Source: CAD feature listing. Evaluate the final solid. Frame: model axes, mm. Round coordinates to 2 decimals unless told otherwise and drop trailing zeros. Loops run counter-clockwise (first coordinate to the right, second up) from the corner with the lowest first, then second, coordinate; pieces in that order, holes last. Notation, with made-up numbers: M 57.25,-3 L 67.25,-3 A30 cw 67.25,36 Z; hole C 44.5,-4.75 d2. An arc over 180 degrees is marked long. Answer as a JSON object with one key per item and string values.
from build123d import *

# Parameters (mm, degrees)
KEYED_BACK_DEPTH   = 0.7
CUP_BLANK_SKETCH_R = 3.8
CUP_BLANK_DEPTH    = 3.3


with BuildPart() as part:
    # Keyed Back Sketch → Keyed Back (new body)
    with BuildSketch(Plane(origin=(0, -97, 0), x_dir=(-1, 0, 0), z_dir=(0, -1, 0))):
        with BuildLine():
            Line((29.790988145, 11.23573341), (33.83079012, 13.568114168))
            ThreePointArc((33.83079012, 13.568114168), (28.410889132, 18.290896534), (29.790988145, 11.23573341))
        make_face()
    extrude(amount=KEYED_BACK_DEPTH)

    # Cup Blank Sketch → Cup Blank (add)
    with BuildSketch(Plane(origin=(0, -97.7, 0), x_dir=(-1, 0, 0), z_dir=(0, -1, 0))):
        with Locations(Location((30.310889132, 15, 0), (0, 0, 262.136353638))):
            Circle(CUP_BLANK_SKETCH_R)
    extrude(amount=CUP_BLANK_DEPTH)

    # Spherical Bearing Seat profile → Spherical Bearing Seat (revolve, cut)
    with BuildSketch(Plane(origin=(0, -101, 0), x_dir=(-1, 0, 0), z_dir=(0, -1, 0))):
        with BuildLine():
            Line((30.310889132, 11.9), (30.310889132, 18.1))
            ThreePointArc((30.310889132, 18.1), (27.210889132, 15), (30.310889132, 11.9))
        make_face()
    revolve(axis=Axis((-30.310889132, -101, -25), (0, 0, 1)), mode=Mode.SUBTRACT)

    # Articulation Throat Sketch → Articulation Throat (revolve, cut)
    with BuildSketch(Plane(origin=(-55.559435073, -21.315405316, -26.260716517), x_dir=(0.37694407644157146, 0.1446147852349051, -0.9148768917876727), z_dir=(0.8541721659092646, 0.32770358269776195, 0.4037329227012915))):
        Polygon((-12.308450042, -83.441173866), (-10.724100051, -81.773890115), (-22.767880189, -61.059022025), (-28.981287547, -67.597673951), align=None)
    revolve(axis=Axis((-25.110986143, -106.383086561, -21.631997284), (-0.5199902989343897, 0.5383086561091633, 0.6631997284167648)), mode=Mode.SUBTRACT)


solid = part.part
Item 1: Contact query for a flat-ended pin moving along its axis: pin 1 Ø1.5 at (x, y) = (-30, -98) entering from +Z. Output: stop coordinate, or through.
Answer sheet:
{"pin 1": "stops at z = -11.31"}
Item 2: Pull-direction query (Y, two-part tool) for faces 1 (the flat face through (-29, -97, -16)), 2 (the flat face through (-27.8, -101, -17.1)), 3 (the conical face through (-30.31, -97.53, -14.87)); classes: pulls with the +Y half, pulls with the -Y half, needs draft (parallel to the pull), parting line crosses it, or undercut.
Answer sheet:
{"face 1": "pulls with the +Y half", "face 2": "pulls with the -Y half", "face 3": "undercut"}
Item 3: Line query: probe 1 along Z at (x, y) = (-27.75, -100.8); probe 2 along Z at (x, y) = (-28.5, -99.25); probe 3 along X at (y, z) = (-100.5, -15.25). Output: solid intervals per line, ascending. Write a range as from..to.
Answer sheet:
{"probe 1": "z = -17.81..-16.74, -13.26..-12.19", "probe 2": "z = -18.34..-16.81, -13.19..-11.66", "probe 3": "x = -34.1..-33.64, -27.26..-26.52"}
Item 4: Section A-A on z = -17.75. Return the cut outline in (x, y).
Answer sheet:
{"outline": "M -32.93,-101 L -31.74,-101 A1.43 cw -28.88,-101 L -27.69,-101 L -27.69,-97 L -32.93,-97 Z"}
